CAD build for the part. Positions are in the model's coordinates, mm. Face numbers are marked on the shaded views. A direction names the side the tool comes from. Give positions to 0.01 mm unless a question says otherwise; leave off trailing zeros. Loops run counter-clockwise (first coordinate to the right, second up) from the corner with the lowest first, then second, coordinate; pieces in that order, holes last.
Autodesk Inventor part; units mm, degrees
ref_plane "Flange Pattern Plane" through (31.75, 7.5406, -4.5466) normal (0, 1, 0) x (1, 0, 0)
ref_plane "YZ Plane" through (0, 0, 0) normal (1, 0, 0) x (0, 1, 0)
ref_plane "XZ Plane" through (0, 0, 0) normal (0, 1, 0) x (-1, 0, 0)
sketch "Sketch1" plane through (0, 0, 0) normal (0, 1, 0) x (-1, 0, 0)
  line L0 (-31.75, 0) -> (31.75, 0)
  line L1 (31.75, 0) -> (31.75, -25.4)
  line L2 (31.75, -25.4) -> (-31.75, -25.4)
  line L3 (-31.75, -25.4) -> (-31.75, 0)
  line L4 (31.75, 0) -> (-31.75, -25.4) construction
  point P0 (0, 0)
  point P1 (0, 0)
  dimension "d0" = 63.5
  dimension "d1" = 25.4
extrude "Plate1" add sketch "Sketch1" along normal blind 1.1906
sketch "Sketch2" plane through (30.5594, 0, -25.4) normal (1, 0, 0) x (0, 1, 0)
  line L0 (0, 25.4) -> (0, 0)
  line L1 (0, 0) -> (13.8906, 0)
  line L2 (13.8906, 0) -> (13.8906, 25.4)
  line L3 (13.8906, 25.4) -> (0, 25.4)
edge flange "Flanges" height 12.7 angle 90 thickness 1.1906 bend radius 0.7937 thickness toward (1, 0, 0) relief tear relief width 1.1906 relief depth 0.5953 corner gap 1.1906 corner form 0 edges at (31.75, 1.1906, -12.7) (-31.75, 1.1906, -12.7) wall of the first edge with corners at (30.5594, 0, 0) (30.5594, 0, -25.4) (30.5594, 13.8906, -25.4) (30.5594, 13.8906, 0)
bend "Bend1"
corner "Corner1"
sketch "Sketch3" plane through (31.75, 1.9844, -25.4) normal (1, 0, 0) x (0, 0, -1)
  line L0 (-20.8534, 7.8676) -> (-17.2466, 7.8676)
  line L1 (-16.7386, 7.3596) -> (-16.7386, 3.7528)
  line L2 (-17.2466, 3.2448) -> (-20.8534, 3.2448)
  line L3 (-21.3614, 3.7528) -> (-21.3614, 7.3596)
  arc A0 (-20.8534, 7.8676) -> (-21.3614, 7.3596) centre (-20.8534, 7.3596) ccw
  arc A1 (-16.7386, 7.3596) -> (-17.2466, 7.8676) centre (-17.2466, 7.3596) ccw
  arc A2 (-17.2466, 3.2448) -> (-16.7386, 3.7528) centre (-17.2466, 3.7528) ccw
  arc A3 (-21.3614, 3.7528) -> (-20.8534, 3.2448) centre (-20.8534, 3.7528) ccw
  line L4 (-25.4, 0) -> (-25.4, 11.9062) construction
  line L5 (-25.4, 11.9062) -> (0, 11.9063) construction
  line L6 (-20.8534, 7.3596) -> (-17.2466, 3.7528) construction
  point P0 (-25.4, -1.9844)
  point P1 (-16.7386, 3.2448)
  point P2 (-21.3614, 3.2448)
  point P3 (-19.05, 5.5562)
  dimension "d16" = 4.6228
  dimension "d17" = 0.508
  dimension "d20" = 6.35
  dimension "d21" = 6.35
extrude "Flange Stamp" cut sketch "Sketch3" against normal blind 1.1906
sketch "Sketch7" plane through (31.75, 1.9844, 0) normal (1, 0, 0) x (0, 0, -1)
  arc A0 (4.5466, 7.8676) -> (4.0386, 7.3596) centre (4.5466, 7.3596) ccw construction
  arc A1 (8.1534, 3.2448) -> (8.6614, 3.7528) centre (8.1534, 3.7528) ccw construction
  circle A2 centre (6.35, 5.5563) radius 2.1844
  line L0 (4.5466, 7.3596) -> (8.1534, 3.7528) construction
  point P0 (0, -1.9844)
  dimension "d46" = 4.3688
surface extrude "Flange Circle" sketch "Sketch7" against normal up to surface (1.1906 mm away) shown yes curves A2
ref_plane "Flange Pattern Plane" through (31.75, 7.5406, -4.5466) normal (0, 1, 0) x (1, 0, 0)
sketch "Flange Pattern Sketch" plane through (31.75, 7.5406, -4.5466) normal (0, 1, 0) x (1, 0, 0)
  line L0 (0, 3.6068) -> (0, 0) construction
  line L1 (-76.2822, -4.5466) -> (13.1932, -4.5466) construction
  line L2 (0, 0) -> (-1.1906, 0) construction
  point P0 (-31.75, -4.5466)
  point P1 (0, 1.8034)
  point P2 (0, 14.5034)
  dimension "d131" = 12.7
  dimension "d134" = 12.7
pattern_sketch "Flange Pattern" of "Flange Circle", "Flange Stamp" from (31.75, 7.5406, -6.35) copies at (31.75, 7.5406, -19.05)
sketch "Sketch8" plane through (0, 0, 0) normal (0, -1, 0) x (1, 0, 0)
  line L0 (29.7656, 0) -> (-29.7656, 0) construction
  line L1 (27.2034, -4.0386) -> (23.5966, -4.0386)
  line L2 (23.0886, -4.5466) -> (23.0886, -8.1534)
  line L3 (23.5966, -8.6614) -> (27.2034, -8.6614)
  line L4 (27.7114, -8.1534) -> (27.7114, -4.5466)
  arc A0 (27.7114, -4.5466) -> (27.2034, -4.0386) centre (27.2034, -4.5466) ccw
  arc A1 (27.2034, -8.6614) -> (27.7114, -8.1534) centre (27.2034, -8.1534) ccw
  arc A2 (23.0886, -8.1534) -> (23.5966, -8.6614) centre (23.5966, -8.1534) ccw
  arc A3 (23.5966, -4.0386) -> (23.0886, -4.5466) centre (23.5966, -4.5466) ccw
  line L5 (27.2034, -4.5466) -> (23.5966, -8.1534) construction
  line L6 (31.75, 0) -> (31.75, -25.4) construction
  point P0 (0, 0)
  point P1 (23.0886, -8.6614)
  point P2 (27.7114, -8.6614)
  point P3 (25.4, -6.35)
  dimension "d49" = 4.6228
  dimension "d50" = 0.508
  dimension "d51" = 6.35
  dimension "d52" = 6.35
extrude "Body Stamp" cut sketch "Sketch8" against normal blind 1.1906
sketch "Sketch9" plane through (0, 0, 0) normal (0, -1, 0) x (1, 0, 0)
  arc A0 (27.7114, -4.5466) -> (27.2034, -4.0386) centre (27.2034, -4.5466) ccw construction
  arc A1 (23.0886, -8.1534) -> (23.5966, -8.6614) centre (23.5966, -8.1534) ccw construction
  line L0 (27.2034, -4.5466) -> (23.5966, -8.1534) construction
  circle A2 centre (25.4, -6.35) radius 2.1844
  point P0 (0, 0)
  dimension "d55" = 4.3688
surface extrude "Body Circle" sketch "Sketch9" against normal up to surface (1.1906 mm away) shown yes curves A2
sketch "Body Pattern Sketch" plane through (0, 0, 0) normal (0, -1, 0) x (1, 0, 0)
  line L0 (29.7656, 0) -> (-29.7656, 0) construction
  line L1 (31.75, 0) -> (31.75, -25.4) construction
  circle A0 centre (25.4, -6.35) radius 2.1844 construction
  point P0 (0, 0)
  point P1 (25.4, -19.05)
  dimension "d62" = 12.7
  dimension "d65" = 12.7
  dimension "d139" = 12.7
pattern_sketch "Body Pattern" of "Body Stamp", "Body Circle" from (25.4, 0, -6.35) copies at (25.4, 0, -19.05)
sketch "Arc Length" plane through (30.5594, 1.9844, 0) normal (0, 0, 1) x (1, 0, 0)
  line L0 (0, 0) -> (1.1906, 0) construction
  arc A0 (-0.7938, -0.7938) -> (0, 0) centre (-0.7938, 0) ccw construction
  line L1 (-0.7938, -1.9844) -> (-0.7938, -0.7938) construction
  arc A1 (-0.7938, -1.9844) -> (1.1906, 0) centre (-0.7938, 0) ccw construction
  point P0 (-30.5594, -1.9844)
  dimension "d85" = 3.117
  dimension "d92" = 1.2468
sketch "Sketch13" plane through (31.75, 13.8906, 0) normal (1, 0, 0) x (0, 0, -1)
  line L0 (0, 0) -> (25.4, 0) construction
  line L1 (62.4078, 0) -> (63.4238, -1.016)
  line L2 (63.4238, -1.016) -> (64.4398, 0)
  line L3 (62.4078, 0) -> (64.4398, 0)
  line L4 (25.4, -11.9063) -> (0, -11.9063) construction
  line L5 (63.4238, -10.8903) -> (61.3168, -12.9972)
  line L6 (61.3168, -12.9972) -> (63.4238, -15.1042)
  line L7 (63.4238, -15.1042) -> (65.5308, -12.9972)
  line L8 (65.5308, -12.9972) -> (63.4238, -10.8903)
  line L9 (63.4238, -10.8903) -> (63.4238, -15.1042) construction
  line L10 (63.4238, -1.016) -> (63.4238, -10.8903) construction
  line L11 (0, -11.9063) -> (25.4, -11.9063) construction
  point P0 (0, -13.8906)
  dimension "d86" = 4.2139
  dimension "d88" = 1.016
  dimension "d91" = 1.016
  dimension "d102" = 63.4238
feature "Notch" [suppressed]
mirror "Notch Mirror" [suppressed]
pattern_linear "Notch Pattern" [suppressed]
chamfer "End Chamfer" distance 1.016 angle 45 4 edges at (-31.1547, 13.8906, -25.4) (31.1547, 13.8906, -25.4) (-31.1547, 13.8906, 0) (31.1547, 13.8906, 0)
sketch "Sketch14" plane through (-31.75, 1.9844, 419.1) normal (1, 0, 0) x (0, 0, -1)
  line L0 (419.1, 11.9063) -> (444.5, 11.9063) construction
  line L1 (419.1, 0) -> (419.1, 11.9063) construction
  line L2 (419.1, -1.9844) -> (444.5, -1.9844) construction
  line L3 (419.1, 11.9063) -> (444.5, 11.9063)
  line L4 (444.5, 11.9063) -> (444.5, -1.9844)
  line L5 (444.5, -1.9844) -> (419.1, -1.9844)
  line L6 (419.1, -1.9844) -> (419.1, 11.9063)
  point P0 (382.0521, -1.9844)
extrude "Half Cut" cut sketch "Sketch14" along normal blind 50.8
equation "\"d1\" = 1.27 * Length"
equation "\"d18\" = Thickness"
equation "\"d53\" = Thickness"
equation "\"d89\" = Thickness"
equation "\"d2\" = Thickness"
equation "\"d3\" = BendReliefWidth"
equation "\"d4\" = BendReliefDepth"
equation "\"d5\" = MinimumRemnant"
equation "\"d6\" = TransitionRadius"
equation "\"d10\" = CornerReliefSize"
equation "\"d11\" = GapSize"
equation "\"d12\" = JacobiRadiusSize"
equation "\"BendRadius\" = Thickness"
equation "\"BendReliefWidth\" = Thickness"
equation "\"BendReliefDepth\" = 0.5 * Thickness"
equation "\"CornerReliefSize\" = 4 * Thickness"
equation "\"MinimumRemnant\" = 2 * Thickness"
equation "\"TransitionRadius\" = BendRadius"
equation "\"JacobiRadiusSize\" = BendRadius"
equation "\"GapSize\" = Thickness"
properties part number "Alu C 1x3x1x35"
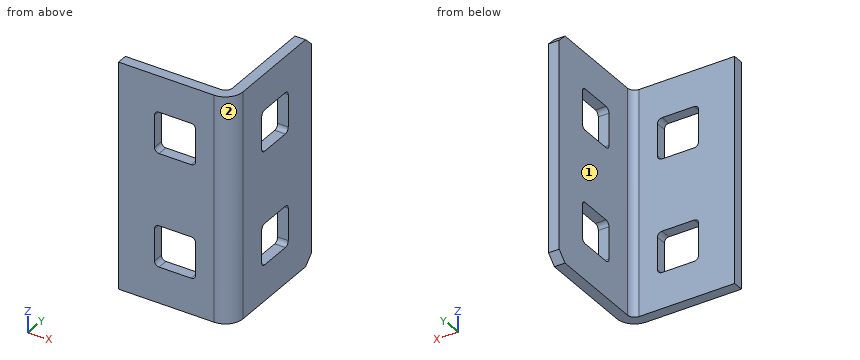
1. Saw through at C-C, the plane z = -6.25. List the corners of the cut face in (x, y).
Responses:
outline: (19.05, 0) - (23.09, 0) - (23.09, 1.19) - (19.05, 1.19) - close; (27.71, 0) - (29.77, 0) arc R1.98 ccw to (31.75, 1.98) - (31.75, 5.23) - (30.56, 5.23) - (30.56, 1.98) arc R0.79 cw to (29.77, 1.19) - (27.71, 1.19) - close; (30.56, 9.85) - (31.75, 9.85) - (31.75, 13.89) - (30.56, 13.89) - close
2. Probe line 1 along X through (y, z) = (5, -7.25); line 2 along Y through (x, z) = (28.25, -2.25); line 3 along X through (y, z) = (1, -9.5). List the from-to ranges inside material, lowest first.
Responses:
line 1: x = 30.56 to 31.75
line 2: y = 0 to 1.19
line 3: x = 19.05 to 31.49
3. Saw through at B-B, the plane y = 6. List the corners of the cut face in (x, z), and give its area (3 significant figures).
Responses:
outline: (30.56, -25.4) - (31.75, -25.4) - (31.75, -21.36) - (30.56, -21.36) - close; (30.56, -16.74) - (31.75, -16.74) - (31.75, -8.66) - (30.56, -8.66) - close; (30.56, -4.04) - (31.75, -4.04) - (31.75, 0) - (30.56, 0) - close
area: 19.2 mm2
4. Drop flat-ended pins along their axis: pin 1 (1 mm diameter, centred on x = 24.5, z = -12, fed in from +Y); pin 2 (2 mm diameter, centred on y = 6, z = -17, fed in from -X); pin 3 (1 mm diameter, centred on x = 31, z = -6.5, fed in from -Y). Give the stop position or say it passes through.
Responses:
pin 1: stops at y = 1.19
pin 2: stops at x = 30.56
pin 3: stops at y = 0.14
5. Saw through at A-A, the plane x = 26.5. List the corners of the cut face in (y, z).
Responses:
outline: (0, -25.4) - (1.19, -25.4) - (1.19, -21.36) - (0, -21.36) - close; (0, -16.74) - (1.19, -16.74) - (1.19, -8.66) - (0, -8.66) - close; (0, -4.04) - (1.19, -4.04) - (1.19, 0) - (0, 0) - close
6. Saw through at D-D, the plane y = 4.5. List the corners of the cut face in (x, z).
Responses:
outline: (30.56, -25.4) - (31.75, -25.4) - (31.75, 0) - (30.56, 0) - close
7. Tool access for the marked faces 1 and 2: list every direction of +Z, -Z, +X, -X, +Y, -Y with a clear straight run to the whole face (end or side of a thin tool).
Responses:
face 1: +Z, -Z, -X, +Y
face 2: +Z, -Z, +X, -Y
